Design review of the part built by this model. Coordinates are the model's own, in mm. A direction names the side the tool comes from. Round coordinates to 2 decimals unless told otherwise and drop trailing zeros. Order: outer loops, then holes, each group sorted by start corner. A loop starts at its lowest first (then second) coordinate and runs counter-clockwise, first axis right, second up. Notation, with made-up numbers: (10.25, 88) - (33.25, 88) arc R28 cw to (33.25, 108) - close; hole circle Ø1 at (70, -33). An arc over 180 degrees is marked (long way). Use CSV: the item, a comma, the result in double quotes. Start each with the question number.
from build123d import *

# Parameters (mm, degrees)
SZKIC2_W                    = 100
SZKIC2_H                    = 23
DODANIE_WYCI_GNI_CIE1_DEPTH = 6
WYTNIJ_WYCI_GNI_CIE1_DEPTH  = 6


with BuildPart() as part:
    # Szkic2 → Dodanie-wyciągnięcie1 (new body)
    with BuildSketch(Plane(origin=(0, 6, 0), x_dir=(1, 0, 0), z_dir=(0, 1, 0))):
        with Locations((34.15799092, -176.577789634)):
            Rectangle(SZKIC2_W, SZKIC2_H)
    extrude(amount=-DODANIE_WYCI_GNI_CIE1_DEPTH)

    # Szkic3 → Wytnij-wyciągnięcie1 (cut)
    with BuildSketch(Plane(origin=(0, 6, 0), x_dir=(1, 0, 0), z_dir=(0, 1, 0))):
        Polygon((64.942961941, -176.577789634), (68.681304934, -183.052789634), (76.15799092, -183.052789634), (79.896333913, -176.577789634), (76.15799092, -170.102789634), (68.681304934, -170.102789634), align=None)
    extrude(amount=-WYTNIJ_WYCI_GNI_CIE1_DEPTH, mode=Mode.SUBTRACT)


solid = part.part
Q1. Tool access review of faces 4 (the flat face through (72, 3, 183.053)), 5 (the flat face through (33, 3, 188.078)): name each direction out of +Z, -Z, +X, -X, +Y, -Y from which nothing blocks a thin tool from reaching the whole face with its end or side.
Q2. The part is to be moulded in two halves that separate along Z. For faces 1 (the flat face through (33, 3, 165.078)), 2 (the flat face through (66.84, 3.04, 173.29)), 3 (the flat face through (84.158, 3, 177)), say which applies: +Z half, -Z half, draft (parallel to the pull), parting line (faces both ways), or undercut.
Q3. For L1, parallel to Z at x = 75, y = 2.7; L2, parallel to X at y = 1.1, z = 174.75; L3, parallel to X at y = 2.3, z = 181.5, list the stretches that pass through material, from the lowest coordinate up. Write a range as [from, to].
Q4. Take a section at A-A (y = 3.3). State the section outline as (x, z) points.
Q5. Take a section at B-B (z = 174.75). State the section outline as (x, y) points, plus the area to 3 significant figures.
Findings below:
1,face 4,"+Y, -Y"
1,face 5,"+Z, +X, -X, +Y, -Y"
2,face 1,"-Z half"
2,face 2,"undercut"
2,face 3,"draft"
3,L1,"z = [165.08, 170.1], [183.05, 188.08]"
3,L2,"x = [-15.84, 66], [78.84, 84.16]"
3,L3,"x = [-15.84, 67.78], [77.05, 84.16]"
4,outline,"(-15.84, 165.08) - (84.16, 165.08) - (84.16, 188.08) - (-15.84, 188.08) - close; hole (64.94, 176.58) - (68.68, 170.1) - (76.16, 170.1) - (79.9, 176.58) - (76.16, 183.05) - (68.68, 183.05) - close"
5,outline,"(-15.84, 0) - (66, 0) - (66, 6) - (-15.84, 6) - close; (78.84, 0) - (84.16, 0) - (84.16, 6) - (78.84, 6) - close"
5,area,"523 mm^2"
